Check sheet for the modelled part. Datum: model origin and axes. Units: mm. Face numbers are marked on the shaded views. A direction names the side the tool comes from. Coordinates: 2 decimals unless noted, no trailing zeros. Loops run counter-clockwise (first coordinate to the right, second up) from the corner with the lowest first, then second, coordinate; pieces in that order, holes last.
from build123d import *

# Parameters (mm, degrees)
SKETCH1_W           = 40
SKETCH1_H           = 40.4
BOSS_EXTRUDE1_DEPTH = 20
SKETCH2_W           = 54.5
SKETCH2_H           = 19
BOSS_EXTRUDE2_DEPTH = 2
SKETCH3_R           = 3
CUT_EXTRUDE1_DEPTH  = 60.284504721
FILLET1_R           = 1
SKETCH4_R           = 2.5
BOSS_EXTRUDE3_DEPTH = 6.223
SKETCH5_W           = 6
SKETCH5_H           = 2.5
BOSS_EXTRUDE4_DEPTH = 6


with BuildPart() as part:
    # Sketch1 → Boss-Extrude1 (new body)
    with BuildSketch(Plane.XY):
        with Locations((20, 20.2)):
            Rectangle(SKETCH1_W, SKETCH1_H)
    extrude(amount=BOSS_EXTRUDE1_DEPTH)

    # Sketch2 → Boss-Extrude2 (add)
    with BuildSketch(Plane(origin=(0, 27.7, 0), x_dir=(-1, 0, 0), z_dir=(0, -1, 0))):
        with Locations((-20, -10)):
            Rectangle(SKETCH2_W, SKETCH2_H)
    extrude(amount=-BOSS_EXTRUDE2_DEPTH)

    # Sketch3 → Cut-Extrude1 (cut, through all)
    with BuildSketch(Plane(origin=(0, 29.7, 0), x_dir=(1, 0, 0), z_dir=(0, 1, 0))):
        with Locations((-4.75, -15)):
            Circle(SKETCH3_R)
        with Locations((-4.75, -5)):
            Circle(SKETCH3_R)
        with Locations((44.75, -5)):
            Circle(SKETCH3_R)
        with Locations((44.75, -15)):
            Circle(SKETCH3_R)
    extrude(amount=-CUT_EXTRUDE1_DEPTH, mode=Mode.SUBTRACT)

    # Fillet1
    fillet1_edges = [part.edges().sort_by_distance(p)[0] for p in [
        (-7.25, 28.7, 19.5),
        (47.25, 28.7, 0.5),
        (-7.25, 28.7, 0.5),
        (47.25, 28.7, 19.5),
    ]]
    fillet(fillet1_edges, radius=FILLET1_R)

    # Sketch4 → Boss-Extrude3 (add)
    with BuildSketch(Plane(origin=(0, 40.4, 0), x_dir=(1, 0, 0), z_dir=(0, 1, 0))):
        with Locations(Location((30.03, -10, 0), (0, 0, 90))):
            Circle(SKETCH4_R)
    extrude(amount=BOSS_EXTRUDE3_DEPTH)

    # Sketch5 → Boss-Extrude4 (add)
    with BuildSketch(Plane(origin=(40, 0, 0), x_dir=(0, 0, -1), z_dir=(1, 0, 0))):
        with Locations((-10, 6.25)):
            Rectangle(SKETCH5_W, SKETCH5_H)
    extrude(amount=BOSS_EXTRUDE4_DEPTH)


solid = part.part
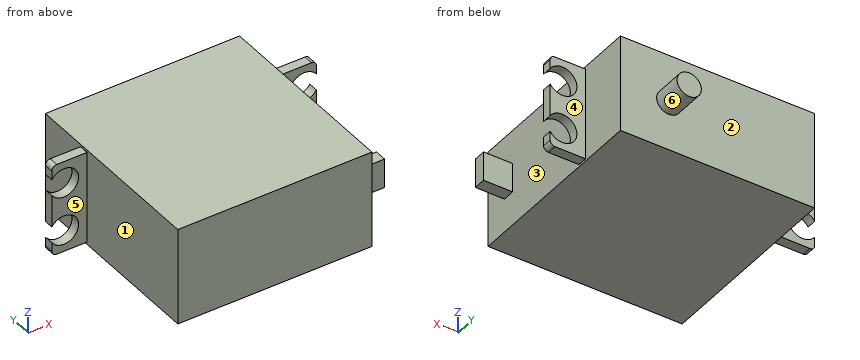
(1) Gauge pin test, flat ends, axial feed: P1, Ø3.5, axis at x = 44.75, z = 15, coming from the -Y side; P2, Ø3, axis at x = 43.5, y = 6.5, coming from the -Z side; P3, Ø2, axis at x = 45, z = 9, coming from the +Y side; P4, Ø6.5, axis at x = 44.5, z = 11.5, coming from the -Y side. Record the tip position at first contact, or that the pin passes through.
(2) Section check B-B, the plane z = 10. Enter the section's corners in (x, y), plus the area to 3 significant figures.
(3) Section check D-D, the plane z = 5. Enter the section's corners in (x, y).
(4) Set-up check for the marked faces 4, 5 and 6: record each of +Z, -Z, +X, -X, +Y, -Y from which the full face is reachable in a straight line by a thin tool's end or side.
(5) Section check C-C, the plane x = 30.03. Enter the section's corners in (y, z), plus the area to 3 significant figures.
(6) Scan lines: line 1 along Z through (x, y) = (44.75, 28.2); line 2 along Y through (x, z) = (-1.5, 4.5); line 3 along X through (y, z) = (9.5, 15.75). Record each from-to range of solid material in increasing order.
(7) Section check A-A, the plane x = -4.75. Enter the section's corners in (y, z), plus the area to 3 significant figures.
(8) Draft check along Y on the marked faces 1, 2 and 3. Enter one of: pulls with the +Y half, pulls with the -Y half, needs draft (parallel to the pull), parting line crosses it, or undercut.
Determined:
1. P1: passes through
1. P2: stops at z = 7
1. P3: stops at y = 29.7
1. P4: stops at y = 5
2. outline: (-7.25, 27.7) - (0, 27.7) - (0, 0) - (40, 0) - (40, 5) - (46, 5) - (46, 7.5) - (40, 7.5) - (40, 27.7) - (47.25, 27.7) - (47.25, 29.7) - (40, 29.7) - (40, 40.4) - (32.53, 40.4) - (32.53, 46.62) - (27.53, 46.62) - (27.53, 40.4) - (0, 40.4) - (0, 29.7) - (-7.25, 29.7) - close
2. area: 1,690 mm2
3. outline: (-1.75, 27.7) - (0, 27.7) - (0, 0) - (40, 0) - (40, 27.7) - (41.75, 27.7) - (41.75, 29.7) - (40, 29.7) - (40, 40.4) - (0, 40.4) - (0, 29.7) - (-1.75, 29.7) - close
4. face 4: +Z, -Z, +X, +Y
4. face 5: +Z, -Z, -X, -Y
4. face 6: +Y
5. outline: (0, 0) - (40.4, 0) - (40.4, 7.5) - (46.62, 7.5) - (46.62, 12.5) - (40.4, 12.5) - (40.4, 20) - (0, 20) - close
5. area: 839 mm2
6. line 1: z = 0.5 to 2, 8 to 12, 18 to 19.5
6. line 2: y = 27.7 to 29.7
6. line 3: x = 0 to 40
7. outline: (27.7, 0.5) - (29.7, 0.5) - (29.7, 2) - (27.7, 2) - close; (27.7, 8) - (29.7, 8) - (29.7, 12) - (27.7, 12) - close; (27.7, 18) - (29.7, 18) - (29.7, 19.5) - (27.7, 19.5) - close
7. area: 14.0 mm2
8. face 1: needs draft
8. face 2: pulls with the +Y half
8. face 3: undercut
